Input: part model. Units: mm. Frame: model coordinates. A direction names the side the tool comes from. Coordinates: 2 decimals unless noted, no trailing zeros. Order: outer loops, then holes, each group sorted by start corner. A loop starts at its lowest first (then second) coordinate and runs counter-clockwise, first axis right, second up.
from build123d import *

# Parameters (mm, degrees)
SKETCH1_R           = 6.875
SKETCH1_R_2         = 6.25
SKETCH1_R_3         = 6.35
SKETCH1_R_4         = 7
SKETCH1_R_5         = 5
SKETCH1_R_6         = 1.5
BOSS_EXTRUDE1_DEPTH = 5
CUT_EXTRUDE1_START  = -5
SKETCH6_R           = 10
CUT_EXTRUDE1_DEPTH  = 1.5
CUT_EXTRUDE2_DEPTH  = 5


with BuildPart() as part:
    # Sketch1 → Boss-Extrude1 (new body)
    with BuildSketch(Plane.XY):
        Polygon((-74.139483312, 85.643418081), (85.860516688, 85.643418081), (140.860516688, -94.356581919), (-74.139483312, -94.356581919), align=None)
        with Locations((-37.139483312, 64.393418081)):
            Circle(SKETCH1_R, mode=Mode.SUBTRACT)
        with Locations((-37.139483312, 43.143418081)):
            Circle(SKETCH1_R, mode=Mode.SUBTRACT)
        with Locations((-37.139483312, 21.893418081)):
            Circle(SKETCH1_R, mode=Mode.SUBTRACT)
        with Locations((-37.139483312, 0.643418081)):
            Circle(SKETCH1_R, mode=Mode.SUBTRACT)
        with Locations((-37.139483312, -20.606581919)):
            Circle(SKETCH1_R, mode=Mode.SUBTRACT)
        with Locations((5.360516688, 52.643418081)):
            Circle(SKETCH1_R_2, mode=Mode.SUBTRACT)
        with Locations((5.360516688, 19.643418081)):
            Circle(SKETCH1_R_2, mode=Mode.SUBTRACT)
        with Locations((5.360516688, -13.356581919)):
            Circle(SKETCH1_R_2, mode=Mode.SUBTRACT)
        with Locations(Location((47.860516688, -13.356581919, 0), (0, 0, 180))):
            Circle(SKETCH1_R_2, mode=Mode.SUBTRACT)
        with Locations(Location((47.860516688, 19.643418081, 0), (0, 0, 180))):
            Circle(SKETCH1_R_2, mode=Mode.SUBTRACT)
        with Locations(Location((47.860516688, 52.643418081, 0), (0, 0, 180))):
            Circle(SKETCH1_R_2, mode=Mode.SUBTRACT)
        with Locations((-37.139483312, -45.356581919)):
            Circle(SKETCH1_R_3, mode=Mode.SUBTRACT)
        with Locations((5.360516688, -45.356581919)):
            Circle(SKETCH1_R_3, mode=Mode.SUBTRACT)
        with Locations((47.860516688, -45.356581919)):
            Circle(SKETCH1_R_3, mode=Mode.SUBTRACT)
        with Locations((-37.139483312, -74.356581919)):
            Circle(SKETCH1_R, mode=Mode.SUBTRACT)
        with Locations((-15.889483312, -74.356581919)):
            Circle(SKETCH1_R_4, mode=Mode.SUBTRACT)
        with Locations((5.360516688, -74.356581919)):
            Circle(SKETCH1_R, mode=Mode.SUBTRACT)
        with Locations((26.610516688, -74.356581919)):
            Circle(SKETCH1_R, mode=Mode.SUBTRACT)
        with Locations((47.860516688, -74.356581919)):
            Circle(SKETCH1_R, mode=Mode.SUBTRACT)
        with Locations((85.860516688, -71.356581919)):
            Circle(SKETCH1_R_5, mode=Mode.SUBTRACT)
        with Locations((-51.639483312, 80.643418081)):
            Circle(SKETCH1_R_6, mode=Mode.SUBTRACT)
        with Locations((61.247280265, 80.643418081)):
            Circle(SKETCH1_R_6, mode=Mode.SUBTRACT)
        with Locations((85.691724709, 0.643418081)):
            Circle(SKETCH1_R_6, mode=Mode.SUBTRACT)
        with Locations((111.663946931, -84.356581919)):
            Circle(SKETCH1_R_6, mode=Mode.SUBTRACT)
        with Locations((-53.139483312, -54.356581919)):
            Circle(SKETCH1_R_6, mode=Mode.SUBTRACT)
    extrude(amount=BOSS_EXTRUDE1_DEPTH)

    # Sketch6 → Cut-Extrude1 (cut)
    with BuildSketch(Plane.XY.offset(5).offset(CUT_EXTRUDE1_START)):
        with Locations((5.360516688, 52.643418081)):
            Circle(SKETCH6_R)
        with Locations((47.860516688, 52.643418081)):
            Circle(SKETCH6_R)
        with Locations((47.860516688, -45.356581919)):
            Circle(SKETCH6_R)
        with Locations((47.860516688, -13.356581919)):
            Circle(SKETCH6_R)
        with Locations((47.860516688, 19.643418081)):
            Circle(SKETCH6_R)
        with Locations((5.360516688, 19.643418081)):
            Circle(SKETCH6_R)
        with Locations((5.360516688, -13.356581919)):
            Circle(SKETCH6_R)
        with Locations((5.360516688, -45.356581919)):
            Circle(SKETCH6_R)
        with Locations((85.860516688, -71.356581919)):
            Circle(SKETCH6_R)
    extrude(amount=CUT_EXTRUDE1_DEPTH, mode=Mode.SUBTRACT)

    # Sketch3 → Cut-Extrude2 (cut)
    with BuildSketch(Plane.XY):
        with BuildLine():
            Line((-74.139483312, 70.643418081), (-70.639483312, 70.643418081))
            ThreePointArc((-70.639483312, 70.643418081), (-65.336182453, 72.840117222), (-63.139483312, 78.143418081))
            Line((-63.139483312, 78.143418081), (-63.139483312, 85.643418081))
            Line((-63.139483312, 85.643418081), (-74.139483312, 85.643418081))
            Line((-74.139483312, 85.643418081), (-74.139483312, 70.643418081))
        make_face()
        with BuildLine():
            Line((136.277183355, -79.356581919), (133.033163973, -79.356581919))
            ThreePointArc((133.033163973, -79.356581919), (129.014117855, -81.382146123), (128.251406117, -85.817674597))
            Line((128.251406117, -85.817674597), (130.860516688, -94.356581919))
            Line((130.860516688, -94.356581919), (140.860516688, -94.356581919))
            Line((140.860516688, -94.356581919), (136.277183355, -79.356581919))
        make_face()
        with BuildLine():
            Line((75.860516688, 85.643418081), (79.668072784, 73.182325403))
            ThreePointArc((79.668072784, 73.182325403), (81.475394843, 70.624371963), (84.449830639, 69.643418081))
            Line((84.449830639, 69.643418081), (90.749405577, 69.643418081))
            Line((90.749405577, 69.643418081), (85.860516688, 85.643418081))
            Line((85.860516688, 85.643418081), (75.860516688, 85.643418081))
        make_face()
        with BuildLine():
            Line((-74.139483312, -79.356581919), (-70.639483312, -79.356581919))
            ThreePointArc((-70.639483312, -79.356581919), (-65.336182453, -81.553281061), (-63.139483312, -86.856581919))
            Line((-63.139483312, -86.856581919), (-63.139483312, -94.356581919))
            Line((-63.139483312, -94.356581919), (-74.139483312, -94.356581919))
            Line((-74.139483312, -94.356581919), (-74.139483312, -79.356581919))
        make_face()
        with BuildLine():
            Line((-74.139483312, -18.146581919), (-68.139483312, -18.146581919))
            ThreePointArc((-68.139483312, -18.146581919), (-64.603949406, -19.611048014), (-63.139483312, -23.146581919))
            Line((-63.139483312, -23.146581919), (-63.139483312, -24.146581919))
            ThreePointArc((-63.139483312, -24.146581919), (-64.603949406, -27.682115825), (-68.139483312, -29.146581919))
            Line((-68.139483312, -29.146581919), (-74.139483312, -29.146581919))
            Line((-74.139483312, -29.146581919), (-74.139483312, -18.146581919))
        make_face()
        with BuildLine():
            Line((111.83273891, 0.643418081), (116.416072243, -14.356581919))
            Line((116.416072243, -14.356581919), (111.744684333, -14.356581919))
            ThreePointArc((111.744684333, -14.356581919), (107.461496787, -12.944008329), (104.858953022, -9.260555376))
            Line((104.858953022, -9.260555376), (104.675619688, -8.660555376))
            ThreePointArc((104.675619688, -8.660555376), (105.773924591, -2.273394373), (111.561351, 0.643418081))
            Line((111.561351, 0.643418081), (111.83273891, 0.643418081))
        make_face()
    extrude(amount=CUT_EXTRUDE2_DEPTH, mode=Mode.SUBTRACT)


solid = part.part
Item 1: Access query for faces 1 (the face through (-31.1, -43.4, 2.5)), 2 (the face through (-63.139, 82, 2)), 3 (the face through (-64.565, -27.643, 2.465)), 4 (the face through (43, -18, 1.5)). Directions: +Z, -Z, +X, -X, +Y, -Y. A direction counts if a zero-diameter tool reaches every point of the face in a straight line with its end or side. Return the directions, or none.
Response values:
face 1: +Z, -Z
face 2: +Z, -Z, -X, +Y
face 3: +Z, -Z, -X
face 4: -Z
Item 2: Draft query along X for faces 5 (the face through (-71, -29.147, 2)), 6 (the face through (82.175, -67.977, 3.226)), 7 (the face through (54.104, 19.369, 3.226)), 8 (the face through (105.72, -2.35, 2.46)). Return one class per face: pulls with the +X half, pulls with the -X half, needs draft (parallel to the pull), parting line crosses it, or undercut.
Response values:
face 5: needs draft
face 6: undercut
face 7: undercut
face 8: pulls with the +X half
Item 3: Cut plane B-B on x = 46. Count the separate pieces of the cut face and the enclosed holes in it, then the cut area to 3 significant figures.
Response values:
separate pieces: 6
enclosed holes: 0
area: 548 mm2
Item 4: Pin query (flat end, axial travel): pin 1 Ø1.5 at (y, z) = (18.5, 2.5) entering from +X; pin 2 Ø3 at (y, z) = (-40, 2.5) entering from +X; pin 3 Ø1 at (x, z) = (134, 2) entering from -Y. Return the tip coordinate at first contact, or that it passes through.
Response values:
pin 1: stops at x = 106.61
pin 2: stops at x = 124.71
pin 3: stops at y = -79.36
Item 5: Cut plane A-A on x = -20. Return loops of the section in (y, z).
Response values:
outline: (-94.36, 0) - (-80.02, 0) - (-80.02, 5) - (-94.36, 5) - close; (-68.69, 0) - (85.64, 0) - (85.64, 5) - (-68.69, 5) - close
Item 6: Ray query, probe 1 along X at (y, z) = (53, 3.3); probe 2 along X at (y, z) = (17.5, 4.05); probe 3 along Y at (x, z) = (0.5, 3.7). Return the intervals inside material, ascending.
Response values:
probe 1: x = -74.14 to -0.88, 11.6 to 41.62, 54.1 to 95.83
probe 2: x = -74.14 to -42.43, -31.85 to -0.51, 11.23 to 41.99, 53.73 to 106.68
probe 3: y = -94.36 to -79.22, -69.49 to -49.44, -41.27 to -17.29, -9.43 to 15.71, 23.57 to 48.71, 56.57 to 85.64
